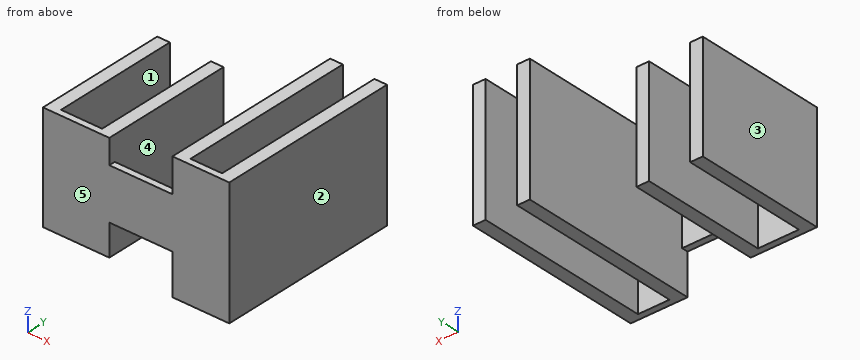
```python
from build123d import *

# Parameters (mm, degrees)
SKETCH1_W           = 2
SKETCH1_H           = 8.5
SKETCH1_H_2         = 20
SKETCH1_H_3         = 17
BOSS_EXTRUDE1_DEPTH = 20
BOSS_EXTRUDE2_DEPTH = 1
SKETCH3_W           = 2
SKETCH3_H           = 20
BOSS_EXTRUDE3_DEPTH = 8


with BuildPart() as part:
    # Sketch1 → Boss-Extrude1 (new body)
    with BuildSketch(Plane(origin=(0, 0, 0), x_dir=(1, 0, 0), z_dir=(0, 1, 0))):
        with Locations((-7.5, 4.25)):
            Rectangle(SKETCH1_W, SKETCH1_H)
        with Locations((-7.5, -4.25)):
            Rectangle(SKETCH1_W, SKETCH1_H)
        with Locations((20, 0)):
            Rectangle(SKETCH1_W, SKETCH1_H_2)
        with Locations((1, 0)):
            Rectangle(SKETCH1_W, SKETCH1_H_3)
        Polygon((14, 10), (14, -10), (12, -10), (12, 0), (12, 10), align=None)
    extrude(amount=BOSS_EXTRUDE1_DEPTH)

    # Sketch2 → Boss-Extrude2 (add)
    with BuildSketch(Plane.XZ):
        Polygon((21, -10), (21, 10), (12, 10), (12, 4.622142766), (2, 4.622142766), (2, 8.5), (-8.5, 8.5), (-8.5, -8.5), (2, -8.5), (2, -3.512828502), (12, -3.512828502), (12, -10), align=None)
    extrude(amount=BOSS_EXTRUDE2_DEPTH)

    # Sketch3 → Boss-Extrude3 (add)
    with BuildSketch(Plane(origin=(0, 20, 0), x_dir=(1, 0, 0), z_dir=(0, 1, 0))):
        with Locations((13, 0)):
            Rectangle(SKETCH3_W, SKETCH3_H)
        with Locations((20, 0)):
            Rectangle(SKETCH3_W, SKETCH3_H)
    extrude(amount=BOSS_EXTRUDE3_DEPTH)


solid = part.part
```
Design review of the part built by this model. Coordinates are the model's own, in mm. Face numbers are marked on the shaded views. A direction names the side the tool comes from. Give positions to 0.01 mm unless a question says otherwise; leave off trailing zeros. Order: outer loops, then holes, each group sorted by start corner. A loop starts at its lowest first (then second) coordinate and runs counter-clockwise, first axis right, second up. Notation, with made-up numbers: (-7, -24.75) -> (43, -24.75) arc R16 cw to (43, -1.75) -> close; hole circle Ø10 at (-27, 83.25). An arc over 180 degrees is marked (long way). Write item = value, one per line. Start each with the question number.
(1) We need section B-B on y = 5. Write out the cut boundary in (x, z).
(2) We need section D-D on z = 0.75. Write out the cut boundary in (x, y).
(3) We need section A-A on z = -4.25. Write out the cut boundary in (x, y).
(4) To check wall thickness, follow line 1 along X through (y, z) = (15.5, 4.25); line 2 along X through (y, z) = (21.25, 0.75); line 3 along Y through (x, z) = (-6.25, -7.5). State the ranges of each line that lie inside material, in increasing order.
(5) For pin 1 (4 mm diameter, centred on x = -5.5, y = 12, fed in from -Z); pin 2 (6.5 mm diameter, centred on x = 5.5, z = 0, fed in from +Y); pin 3 (11.5 mm diameter, centred on x = -5.5, y = 4.5, fed in from +Z), all flat-tipped, find the tip position at first contact; note any pin that passes through.
(6) We need section C-C on y = 25. Write out the cut boundary in (x, z).
(7) Mouldability with a two-part tool opening along X and no side actions: class the marked faces 3, 4 and 5 as +X half, -X half, draft (parallel to the pull), parting line (faces both ways), or undercut.
(8) For the marked faces 1 and 2, list the 3-axis set-ups (+Z, -Z, +X, -X, +Y, -Y) from which the entire face can be reached by the end or side of a thin tool; tool diameter is ignored.
Numbers:
q1.outline = (-8.5, -8.5) -> (-6.5, -8.5) -> (-6.5, 8.5) -> (-8.5, 8.5) -> close; (0, -8.5) -> (2, -8.5) -> (2, 8.5) -> (0, 8.5) -> close; (12, -10) -> (14, -10) -> (14, 10) -> (12, 10) -> close; (19, -10) -> (21, -10) -> (21, 10) -> (19, 10) -> close
q2.outline = (-8.5, -1) -> (21, -1) -> (21, 28) -> (19, 28) -> (19, 0) -> (14, 0) -> (14, 28) -> (12, 28) -> (12, 0) -> (2, 0) -> (2, 20) -> (0, 20) -> (0, 0) -> (-6.5, 0) -> (-6.5, 20) -> (-8.5, 20) -> close
q3.outline = (-8.5, -1) -> (2, -1) -> (2, 20) -> (0, 20) -> (0, 0) -> (-6.5, 0) -> (-6.5, 20) -> (-8.5, 20) -> close; (12, -1) -> (21, -1) -> (21, 28) -> (19, 28) -> (19, 0) -> (14, 0) -> (14, 28) -> (12, 28) -> close
q4.line_1 = -8.5 to -6.5, 0 to 2, 12 to 14, 19 to 21
q4.line_2 = 12 to 14, 19 to 21
q4.line_3 = -1 to 0
q5.pin_1 = -8.5
q5.pin_2 = 0
q5.pin_3 = 8.5
q6.outline = (12, -10) -> (14, -10) -> (14, 10) -> (12, 10) -> close; (19, -10) -> (21, -10) -> (21, 10) -> (19, 10) -> close
q7.face_3 = -X half
q7.face_4 = undercut
q7.face_5 = draft
q8.face_1 = +Z, -Z, +Y
q8.face_2 = +Z, -Z, +X, +Y, -Y
